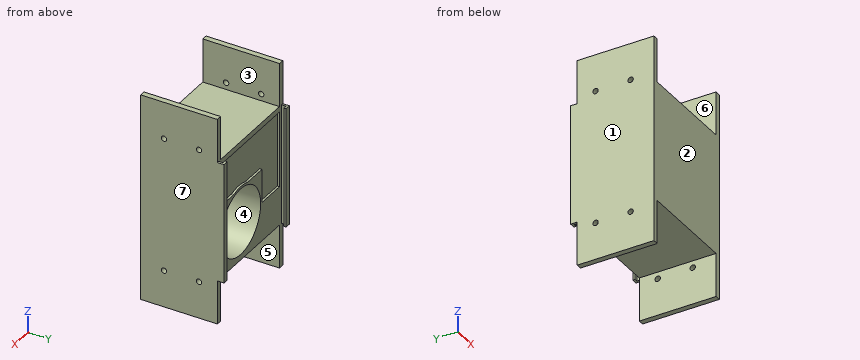
Autodesk Inventor part; units mm, degrees
ref_plane "YZ Plane" through (0, 0, 0) normal (1, 0, 0) x (0, 1, 0)
ref_plane "XZ Plane" through (0, 0, 0) normal (0, 1, 0) x (-1, 0, 0)
ref_plane "XY Plane" through (0, 0, 0) normal (0, 0, 1) x (1, 0, 0)
sketch "Sketch1" plane through (0, 0, 0) normal (0, 1, 0) x (-1, 0, 0)
  line L0 (0, 0) -> (0, -190)
  line L1 (0, -190) -> (100, -190)
  line L2 (100, -190) -> (100, 0)
  line L3 (100, 0) -> (0, 0)
  line L4 (95, -5) -> (95, -185)
  line L5 (95, -185) -> (5, -185)
  line L6 (5, -185) -> (5, -5)
  line L7 (5, -5) -> (95, -5)
  line L8 (95, -5) -> (95, 0)
  line L9 (95, -185) -> (95, -190)
  line L10 (5, -185) -> (5, -190)
  line L11 (5, -5) -> (5, 0)
  line L12 (100, -45) -> (0, -45)
  line L13 (0, -45) -> (0, -145)
  line L14 (0, -145) -> (100, -145)
  line L15 (100, -145) -> (100, -45)
  line L16 (100, -40) -> (0, -40)
  line L17 (100, -150) -> (0, -150)
  point P0 (100, -95)
  point P1 (100, -95)
  point P2 (5, -150)
  point P3 (95, -150)
  point P4 (95, -40)
  point P5 (5, -40)
  point P6 (95, -145)
  point P7 (5, -145)
  point P8 (5, -45)
  point P9 (95, -45)
  dimension "d0" = 190
  dimension "d1" = 100
  dimension "d2" = 100
  dimension "d3" = 5
  dimension "d4" = 5
extrude "Extrusion1" add sketch "Sketch1" along normal blind 65 contours L3 L11 L6 L16 L0 | L16 L6 L12 L0 | L12 L6 L14 L0 | L3 L2 L16 L4 L8 | L14 L6 L17 L0 | L16 L2 L12 L4 | L17 L6 L10 L1 L0 | L12 L2 L14 L4 | L14 L2 L17 L4 | L17 L2 L1 L9 L4
extrude "Extrusion2" add sketch "Sketch1" against normal blind 5 contours L3 L11 L6 L16 L0 | L16 L6 L12 L0 | L12 L6 L14 L0 | L16 L4 L12 L6 | L3 L2 L16 L4 L8 | L14 L6 L17 L0 | L12 L4 L14 L6 | L16 L2 L12 L4 | L17 L6 L10 L1 L0 | L14 L4 L17 L6 | L12 L2 L14 L4 | L14 L2 L17 L4 | L17 L2 L1 L9 L4
extrude "Extrusion3" add sketch "Sketch1" along normal blind 65 contours L14 L4 L17 L6
extrude "Extrusion5" add sketch "Sketch1" along normal blind 65 contours L16 L4 L12 L6
sketch "Sketch2" plane through (0, 0, 0) normal (0, 1, 0) x (1, 0, 0)
  circle A0 centre (-35.6617, 114.4032) radius 30.5
  circle A1 centre (-35.6617, 114.4032) radius 32.5
  point P0 (0, 0)
  dimension "d11" = 61
  dimension "d12" = 65
extrude "Extrusion4" add sketch "Sketch2" along normal blind 65
sketch "Sketch3" plane through (-5, 0, -103.6278) normal (-1, 0, 0) x (0, 0, 1)
  line L0 (-41.3722, 65) -> (-21.5507, 65)
  line L1 (58.6278, 0) -> (58.6278, 65)
  line L2 (-41.3722, 65) -> (58.6278, 65)
  line L3 (58.6278, 65) -> (58.6278, 62)
  line L4 (58.6278, 62) -> (-41.3722, 62)
  line L5 (-41.3722, 62) -> (-41.3722, 65)
  point P0 (103.6278, 0)
  dimension "d17" = 3
extrude "Extrusion6" add sketch "Sketch3" along normal up to surface (90 mm away)
extrude "Extrusion7" cut sketch "Sketch2" along normal blind 66.5 contours A0
sketch "Sketch4" plane through (0, 65, 0) normal (0, 1, 0) x (1, 0, 0)
  line L0 (-95, 145) -> (-95, 45)
  line L1 (-5, 45) -> (-5, 103.6278)
  line L2 (-95, 45) -> (-5, 45)
  line L3 (-5, 45) -> (-5, 83.6142)
  line L4 (-5, 83.6142) -> (-95, 83.6142)
  line L5 (-95, 83.6142) -> (-95, 45)
  arc A0 (-46.6201, 145) -> (-5, 103.6278) centre (-35.6617, 114.4032) ccw
  line L6 (-95, 83.6142) -> (-68.1617, 83.6142)
  line L7 (-68.1617, 83.6142) -> (-68.1617, 114.4032)
  line L8 (-68.1617, 114.4032) -> (-95, 114.4032)
  line L9 (-95, 114.4032) -> (-95, 83.6142)
  point P0 (0, 0)
  point P1 (-25.2556, 83.6142)
  point P2 (-46.0678, 83.6142)
extrude "Extrusion8" cut sketch "Sketch4" against normal blind 2 contours L8 L7 L4 L0 | L4 A0 L1 L2 L0
sketch "Sketch5" plane through (0, 65, 0) normal (1, 0, 0) x (0, 0, -1)
  circle A0 centre (33.7554, -16.723) radius 5.5293
  circle A1 centre (33.7554, -48.723) radius 5.535
  circle A2 centre (156.2446, -16.723) radius 5.926
  circle A3 centre (156.2446, -48.723) radius 6.0534
  line L0 (33.7554, -16.723) -> (33.7554, -48.723)
  line L1 (33.7554, -16.723) -> (156.2446, -16.723)
  line L2 (0, 0) -> (190, 0)
  line L3 (0, -70) -> (0, 0)
  line L4 (0, 0) -> (190, 0)
  point P0 (0, -65)
  point P1 (95, -16.723)
  point P2 (33.7554, -32.723)
  point P3 (95, 0)
  dimension "d24" = 16.723
  dimension "d25" = 32
hole "Hole1" at (0, 48.277, -33.7554) at (0, 16.277, -33.7554) at (0, 16.277, -156.2446) at (0, 48.277, -156.2446) direction (-1, 0, 0) diameter 4.917 depth 17.1
ref_plane "Work Plane1" through (-50, 65, 0) normal (1, 0, 0) x (0, 0, -1)
mirror "Mirror1" about plane through (-50, 65, 0) normal (1, 0, 0) of "Hole1"
sketch "Sketch6" plane through (0, 65, 0) normal (0, 1, 0) x (1, 0, 0)
  line L0 (-95, 150) -> (-95, 190)
  line L1 (-95, 150) -> (-100, 150)
  line L2 (-100, 190) -> (-100, 0)
  line L3 (-95, 40) -> (-5, 40)
  line L4 (-95, 40) -> (-100, 40)
  line L5 (-100, 150) -> (-95, 150)
  line L6 (-95, 150) -> (-95, 40)
  line L7 (-95, 40) -> (-100, 40)
  line L8 (-100, 40) -> (-100, 150)
  line L9 (0, 0) -> (0, 190)
  line L10 (-5, 150) -> (0, 150)
  line L11 (0, 150) -> (0, 40)
  line L12 (0, 40) -> (-5, 40)
  line L13 (-5, 40) -> (-5, 150)
extrude "Extrusion9" add sketch "Sketch6" along normal blind 6
sketch "Sketch7" plane through (-100, 65, -40) normal (0, 0, 1) x (1, 0, 0)
  line L0 (5, 0) -> (5, 6)
  line L1 (5, 4) -> (5, 0)
  line L2 (5, 0) -> (2, 0)
  line L3 (2, 0) -> (2, 4)
  line L4 (2, 4) -> (5, 4)
  line L5 (94.9938, 4) -> (97.9938, 4)
  line L6 (97.9938, 4) -> (97.9938, 0)
  line L7 (97.9938, 0) -> (94.9938, 0)
  line L8 (94.9938, 0) -> (94.9938, 4)
  line L9 (5, 0) -> (5, 6)
  line L10 (0, 0) -> (5, 0)
  line L11 (95, 0) -> (100, 0)
  point P0 (100, -65)
  dimension "d35" = 4
  dimension "d36" = 3
  dimension "d37" = 3
  dimension "d38" = 4
  dimension "d39" = 0
  dimension "d40" = 0
extrude "Extrusion10" cut sketch "Sketch7" against normal up to surface (110 mm away)
properties part number "MiddlePart"
For this review, take the finished solid that the model builds, in its own axes (mm). Face numbers are marked on the shaded views. A direction names the side the tool comes from. Round coordinates to 2 decimals unless told otherwise and drop trailing zeros. Write each loop counter-clockwise with the first axis right and the second up, starting at its lowest first coordinate (ties: lowest second). Pieces come first, ordered by that corner, then holes. Notation, with made-up numbers: (-22.5, -37) -> (-8.5, -37) arc R15 ccw to (-8.5, -30) -> close; hole circle Ø6 at (-0.5, 59). An arc over 180 degrees is marked (long way). One line per question, with ' | ' between items. Start each with the question number.
1) Machinability: for the marked faces 4, 5, 6 and 7, which of the approach directions +Z, -Z, +X, -X, +Y, -Y give a long, thin tool a straight path to every point of the face, cutting with its end or side? Answer none if there is none.
2) Mouldability with a two-part tool opening along X and no side actions: class the marked faces 1, 2 and 3 as +X half, -X half, draft (parallel to the pull), parting line (faces both ways), or undercut.
3) Wall thickness on line 1 along X through (y, z) = (24, -115.5); line 2 along Z through (x, y) = (-37, 19); line 3 along Z through (x, y) = (-83.5, 53.5): over which ranges is each line inside the solid? List them lowest first.
4) Add section B-B (y = 33). Write out the cut boundary in (x, z), and give its area (3 significant figures).
5) For pin 1 Ø4 at (x, z) = (-88.5, -75.5) entering from +Y; pin 2 Ø0.6 at (x, y) = (-55, 64) entering from +Z; pin 3 Ø12 at (x, y) = (-28, 32.5) entering from -Z, all flat-tipped, find the tip position at first contact; note any pin that passes through.
6) Add section C-C (x = -59.5). Write out the cut boundary in (y, z), and give its area (3 significant figures).
7) Add section D-D (z = -74.5). Write out the cut boundary in (x, y), and give its area (3 significant figures).
8) Add section A-A (z = -12). Write out the cut boundary in (x, y), and give its area (3 significant figures).
Reported:
1) face 4: +Y | face 5: -Z, +Y, -Y | face 6: +Z, +Y, -Y | face 7: +Z, -Z, +X, +Y, -Y
2) face 1: -X half | face 2: draft | face 3: undercut
3) line 1: x = -100 to -95, -68.14 to -66.14, -5.18 to 0 | line 2: z = -150 to -144.87, -83.93 to -81.93, -45 to -40 | line 3: z = -150 to -145, -45 to -40
4) outline: (-100, -190) -> (-95, -190) -> (-95, -150) -> (-5, -150) -> (-5, -190) -> (0, -190) -> (0, 0) -> (-5, 0) -> (-5, -40) -> (-95, -40) -> (-95, 0) -> (-100, 0) -> close; hole (-95, -145) -> (-46.62, -145) arc R32.5 cw (long way) to (-5, -103.63) -> (-5, -45) -> (-95, -45) -> close; hole circle Ø61 at (-35.66, -114.4); hole (-24.7, -145) -> (-5, -145) -> (-5, -125.18) arc R32.5 cw to start | area: 3,140 mm²
5) pin 1: stops at y = 63 | pin 2: stops at z = -40 | pin 3: stops at z = -150
6) outline: (-5, -150) -> (65, -150) -> (65, -133.43) -> (0, -133.43) -> (0, -95.38) -> (65, -95.38) -> (65, -83.61) -> (63, -83.61) -> (63, -45) -> (65, -45) -> (65, -40) -> (-5, -40) -> close; hole (0, -145) -> (62, -145) -> (62, -136.49) -> (0, -136.49) -> close; hole (0, -92.31) -> (62, -92.31) -> (62, -45) -> (0, -45) -> close | area: 1,690 mm²
7) outline: (-100, -5) -> (0, -5) -> (0, 71) -> (-5, 71) -> (-5, 69) -> (-2.01, 69) -> (-2.01, 65) -> (-5, 65) -> (-5, 63) -> (-95, 63) -> (-95, 65) -> (-98, 65) -> (-98, 69) -> (-95, 69) -> (-95, 71) -> (-100, 71) -> close; hole (-95, 0) -> (-5, 0) -> (-5, 62) -> (-95, 62) -> close | area: 1,280 mm²
8) outline: (-100, -5) -> (-95, -5) -> (-95, 65) -> (-100, 65) -> close; (-5, -5) -> (0, -5) -> (0, 65) -> (-5, 65) -> close | area: 700 mm²
